from build123d import *

# Parameters (mm, degrees)
BOSS_EXTRU_1_DEPTH            = 3
TROU_DE_PASSAGE_D_AXE_3_321_D = 2
TROU_DE_PASSAGE_D_AXE_3_322_D = 2


with BuildPart() as part:
    # Esquisse1 → Boss.-Extru.1 (new body)
    with BuildSketch(Plane.XY):
        with BuildLine():
            Line((0, 44.592200572), (0, -30.407799428))
            ThreePointArc((0, -30.407799428), (3.5, -33.907799428), (7, -30.407799428))
            Line((7, -30.407799428), (7, 44.592200572))
            ThreePointArc((7, 44.592200572), (10.5782573, 56.097095666), (19.122245191, 64.592200572))
            ThreePointArc((19.122245191, 64.592200572), (19.045221408, 69.669224354), (13.968197626, 69.592200572))
            ThreePointArc((13.968197626, 69.592200572), (4.030461038, 58.742480417), (0, 44.592200572))
        make_face()
    extrude(amount=BOSS_EXTRU_1_DEPTH)

    # Trou de passage d'axe 3/321 (through all)
    with Locations(Plane(origin=(16.545221408, 67.092200572, 3), x_dir=(1, 0, 0), z_dir=(0, 0, 1))):
        with Locations((0, 0)):
            Hole(TROU_DE_PASSAGE_D_AXE_3_321_D / 2)

    # Trou de passage d'axe 3/322 (through all)
    with Locations(Plane(origin=(3.5, -30.407799428, 3), x_dir=(1, 0, 0), z_dir=(0, 0, 1))):
        with Locations((0, 0)):
            Hole(TROU_DE_PASSAGE_D_AXE_3_322_D / 2)


solid = part.part
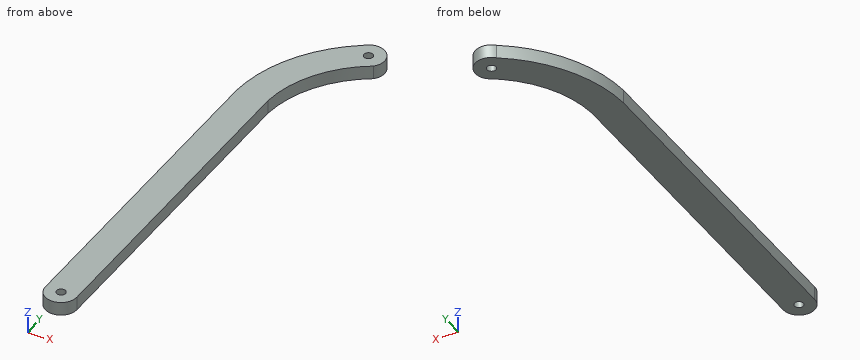
Build history of the part. All positions in model axes, mm. Round coordinates to 2 decimals unless told otherwise and drop trailing zeros. Write each loop counter-clockwise with the first axis right and the second up, starting at its lowest first coordinate (ties: lowest second). Pieces come first, ordered by that corner, then holes. Notation, with made-up numbers: M -34,29.5 L -23,29.5 A18 ccw -23,50.5 Z; hole C -14,-37.5 d8. An arc over 180 degrees is marked long. Answer as a JSON object with one key per item and string values. Group by question number.
(1) Cut at C-C (x = 3.5). Give the cut face in (y, z), and give its area (3 significant figures).
(2) Cut at B-B (z = 2.15). Give the cut face in (x, y), and give its area (3 significant figures).
(3) Flat gauge pins, fed straight in: pin 1 (3 mm diameter, centred on x = 4.5, y = -16, fed in from -Z); pin 2 (0.9 mm diameter, centred on y = -6.5, z = 1.5, fed in from +X). Where does each tip first touch, or does it go through?
(4) Drill centre lines: L1, parallel to X at y = 8.5, z = 0.9; L2, parallel to Y at x = 3.5, z = 1.5; L3, parallel to Y at x = 3.25, z = 1.7. Where is each one in solid material? Low to high.
(5) Cut at A-A (x = 16.5). Give the cut face in (y, z), and give its area (3 significant figures).
(6) Cut at D-D (y = -16.5). Give the cut face in (x, z).
Responses:
{
 "1": {"outline": "M -33.91,0 L -31.41,0 L -31.41,3 L -33.91,3 Z; M -29.41,0 L 57.75,0 L 57.75,3 L -29.41,3 Z", "area": "269 mm2"},
 "2": {"outline": "M 0,-30.41 A3.5 ccw 7,-30.41 L 7,44.59 A25 cw 19.12,64.59 A3.59 ccw 13.97,69.59 A31.99 ccw 0,44.59 Z; hole C 3.5,-30.41 d2; hole C 16.55,67.09 d2", "area": "747 mm2"},
 "3": {"pin 1": "stops at z = 0", "pin 2": "stops at x = 7"},
 "4": {"L1": "x = 0 to 7", "L2": "y = -33.91 to -31.41, -29.41 to 57.75", "L3": "y = -33.9 to -31.38, -29.44 to 57.26"},
 "5": {"outline": "M 62.79,0 L 66.09,0 L 66.09,3 L 62.79,3 Z; M 68.09,0 L 70.68,0 L 70.68,3 L 68.09,3 Z", "area": "17.7 mm2"},
 "6": {"outline": "M 0,0 L 7,0 L 7,3 L 0,3 Z"}
}
